Autodesk Inventor part; units mm, degrees
ref_plane "YZ Plane" through (0, 0, 0) normal (1, 0, 0) x (0, 1, 0)
ref_plane "XZ Plane" through (0, 0, 0) normal (0, 1, 0) x (-1, 0, 0)
ref_plane "XY Plane" through (0, 0, 0) normal (0, 0, 1) x (1, 0, 0)
sketch "Sketch1" plane through (0, 0, 0) normal (0, 0, 1) x (1, 0, 0)
  line L0 (0, 0) -> (0, -43.1) construction
  line L1 (12, 0) -> (12, -30)
  line L2 (12, -30) -> (13.5, -30)
  line L3 (13.5, -30) -> (17.25, -2)
  line L4 (18.25, 2) -> (15, 2)
  line L5 (15, 2) -> (15, 0)
  line L6 (15, 0) -> (12, 0)
  line L7 (17.25, -2) -> (18.25, -2)
  line L8 (18.25, -2) -> (18.25, 2)
  dimension "d1" = 36.5
  dimension "d2" = 24
  dimension "d3" = 30
  dimension "d4" = 2
  dimension "d5" = 1
  dimension "d6" = 30
  dimension "d7" = 27
  dimension "d8" = 2
revolve "Revolution1" add sketch "Sketch1" angle 360 about axis through (0, 0, 0) along (0, -1, 0)
properties part number "002" material "Iron, Cast"
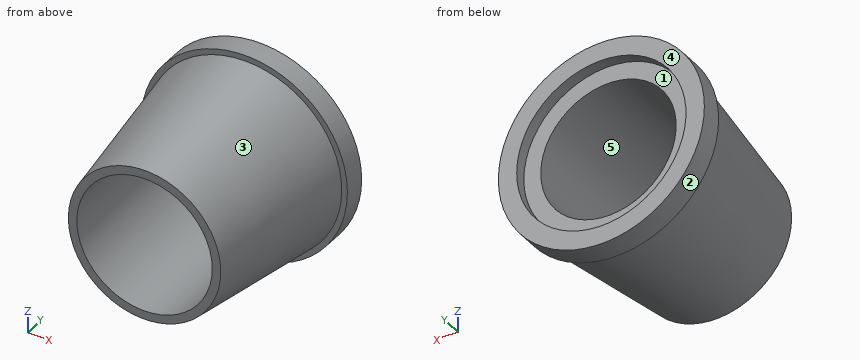
Part model, mm, in its own coordinate system. Face numbers are marked on the shaded views. A direction names the side the tool comes from. Coordinates: 2 decimals unless noted, no trailing zeros. Write each loop counter-clockwise with the first axis right and the second up, starting at its lowest first coordinate (ties: lowest second). Pieces come first, ordered by that corner, then holes.
Item 1: Pin check, flat tips, straight feed: pin 1 (14.5 mm diameter, centred on x = 0, z = 0, fed in from +Y); pin 2 (12 mm diameter, centred on x = 8, y = -10, fed in from -Z); pin 3 (1.5 mm diameter, centred on x = 10, z = -10, fed in from +Y); pin 4 (12 mm diameter, centred on x = 2, y = -22.5, fed in from -Z). Stop position of each tip, or through.
Item 2: Which spindle directions (+Z, -Z, +X, -X, +Y, -Y) get a long thin tool onto all of the face, cutting with end or side? Do the marked faces 1 and 2. Say none if no direction does.
Item 3: Slice it at B-B (x = 0). Write the cut outline in (y, z).
Item 4: Slice it at A-A (z = 0). Write the cut outline in (x, y), and give its area (3 significant figures).
Item 5: Slice it at D-D (y = -27.5). Write the cut outline in (x, z), and give its area (3 significant figures).
Item 6: Probe line 1 (Z direction, x = 0, y = 1.5); line 2 (X direction, y = -12.5, z = 8.5); line 3 (Z direction, x = 0, y = -15). List the from-to ranges inside material, lowest first.
Item 7: Mould opens along Z. For the marked faces 3, 4 and 5 say: released by +Z, released by -Z, zero draft, split by the parting line, or undercut.
Item 8: Slice it at C-C (y = -18). Write the cut outline in (x, z), and give its area (3 significant figures).
Results found:
1. pin 1: passes through
1. pin 2: stops at z = -16.35
1. pin 3: stops at y = 0
1. pin 4: stops at z = -15.27
2. face 1: +Y
2. face 2: +Y, -Y
3. outline: (-30, -13.5) - (-2, -17.25) - (-2, -18.25) - (2, -18.25) - (2, -15) - (0, -15) - (0, -12) - (-30, -12) - close; (-30, 12) - (0, 12) - (0, 15) - (2, 15) - (2, 18.25) - (-2, 18.25) - (-2, 17.25) - (-30, 13.5) - close
4. outline: (-18.25, -2) - (-17.25, -2) - (-13.5, -30) - (-12, -30) - (-12, 0) - (-15, 0) - (-15, 2) - (-18.25, 2) - close; (12, -30) - (13.5, -30) - (17.25, -2) - (18.25, -2) - (18.25, 2) - (15, 2) - (15, 0) - (12, 0) - close
4. area: 227 mm2
5. outline: circle Ø27.67 at (0, 0); hole circle Ø24 at (0, 0)
5. area: 149 mm2
6. line 1: z = -18.25 to -15, 15 to 18.25
6. line 2: x = -13.37 to -8.47, 8.47 to 13.37
6. line 3: z = -15.51 to -12, 12 to 15.51
7. face 3: split by the parting line
7. face 4: zero draft
7. face 5: undercut
8. outline: circle Ø30.21 at (0, 0); hole circle Ø24 at (0, 0)
8. area: 265 mm2
